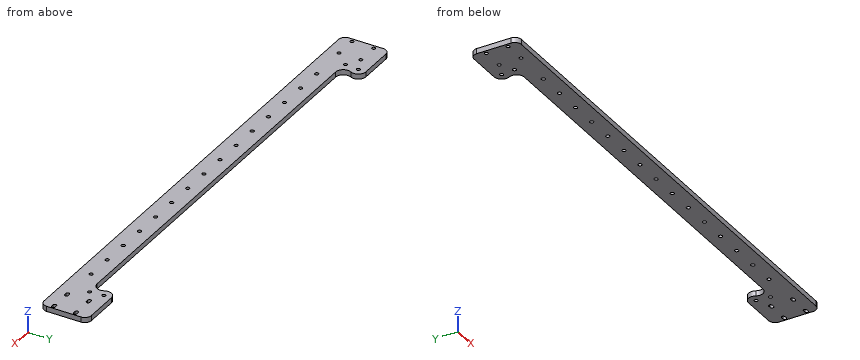
Solid Edge part; units mm, degrees
sketch "Sketch1" plane through (0, 0, 0) normal (0, 0, 1) x (1, 0, 0)
  line L0 (-13.5, 22.7) -> (-13.5, -20.7)
  line L1 (-13.5, -20.7) -> (221, -20.7)
  line L2 (455.5, -20.7) -> (221, -20.7)
  line L3 (455.5, 22.7) -> (455.5, -20.7)
  line L4 (455.5, 22.7) -> (418.43, 22.7)
  arc A0 (418.43, 22.7) -> (412.2867, 12.5) centre (418.43, 15.75) ccw
  arc A1 (412.2867, 12.5) -> (406.1434, 2.3) centre (406.1434, 9.25) cw
  line L5 (406.1434, 2.3) -> (221, 2.3)
  line L6 (35.8566, 2.3) -> (221, 2.3)
  arc A2 (29.7133, 12.5) -> (35.8566, 2.3) centre (35.8566, 9.25) ccw
  arc A3 (23.57, 22.7) -> (29.7133, 12.5) centre (23.57, 15.75) cw
  line L7 (-13.5, 22.7) -> (23.57, 22.7)
extrude "Protrusion1" add sketch "Sketch1" along normal blind 4.7625
hole "Hole_1" at (-10, 10, 4.7625) direction (0, 0, -1) diameter 3.2 end up to next
hole "Hole_5" at (46, -9.2, 4.7625) direction (0, 0, -1) diameter 3.4 end up to next
pattern_linear "Pattern2" count 15 spacing 25 along (1, 0, 0) of "Hole_5"
hole "Hole_6" at (23.57, 15.75, 4.7625) direction (0, 0, -1) diameter 3.242 end up to next
hole "Hole1" at (22.47, 3.33, 4.7625) direction (0, 0, -1) diameter 3.242 end up to next
hole "Hole2" at (418.43, 15.75, 4.7625) direction (0, 0, -1) diameter 3.242 end up to next
hole "Hole3" at (419.53, 3.33, 4.7625) direction (0, 0, -1) diameter 3.242 end up to next
pattern_linear "Pattern5" count 2 spacing 20 along (1, 0, 0) count 2 spacing 20 along (0, -1, 0) of "Hole_1"
sketch "Sketch2" plane through (221, 1, 4.7625) normal (0, 0, 1) x (-1, 0, 0)
  line L0 (-212, -10.6) -> (-210, -10.6)
  arc A0 (-210, -10.6) -> (-210, -7.4) centre (-210, -9) ccw
  line L1 (-210, -7.4) -> (-212, -7.4)
  arc A1 (-212, -7.4) -> (-212, -10.6) centre (-212, -9) ccw
  dimension "D1" = 212
extrude "Cutout1" cut sketch "Sketch2" against normal up to next
pattern_linear "Pattern7" count 2 spacing 20 along (1, 0, 0) count 2 spacing 20 along (0, -1, 0) of "Cutout1"
fillet "Round_2" radius 5.95 4 edges at (-13.5, -20.7, 2.3812) (-13.5, 22.7, 2.3812) (455.5, -20.7, 2.3812) (455.5, 22.7, 2.3812)
properties material "Aluminum, 6061-T6"
Work out the finished part from the listing and answer in its coordinate system (mm). Give positions to 0.01 mm unless a question says otherwise; leave off trailing zeros. Loops run counter-clockwise (first coordinate to the right, second up) from the corner with the lowest first, then second, coordinate; pieces in that order, holes last. Notation, with made-up numbers: (63.5, 0) -> (101.5, 0) arc R34 ccw to (101.5, 33) -> close; hole circle Ø10 at (-21, 75.5). An arc over 180 degrees is marked (long way). Use a Markdown table: item, result. Add a question column.
1. Find the intervals of material crossed by probe 1 along Y at (x, z) = (10, 1.95); probe 2 along X at (y, z) = (15.75, 3.75); probe 3 along Y at (x, z) = (246, 1), in increasing order.
2. Section A-A on x = 329 is taken. Determine the outline of the cut face in (y, z).
3. Flat-ended cylindrical pins translate along their axes: pin 1 Ø1.4 at (x, z) = (247.5, 3) entering from +Y; pin 2 Ø0.6 at (x, z) = (452, 3.5) entering from -Y. Find the tip coordinate at first contact, or state that the pin passes through.
4. Section B-B on z = 2.85 is taken. State how many separate pieces and enclosed holes the cut face has, and give its area (3 significant figures).
Results below:
| question | item | result |
|---|---|---|
| 1 | probe 1 | y = -20.7 to -11.6, -8.4 to 8.4, 11.6 to 22.7 |
| 1 | probe 2 | x = -13.5 to 21.95, 25.19 to 30.52, 411.48 to 416.81, 420.05 to 455.5 |
| 1 | probe 3 | y = -20.7 to -10.9, -7.5 to 2.3 |
| 2 | outline | (-20.7, 0) -> (2.3, 0) -> (2.3, 4.76) -> (-20.7, 4.76) -> close |
| 3 | pin 1 | stops at y = 2.3 |
| 3 | pin 2 | stops at y = -20.3 |
| 4 | separate pieces | 1 |
| 4 | enclosed holes | 27 |
| 4 | area | 12,300 mm^2 |
